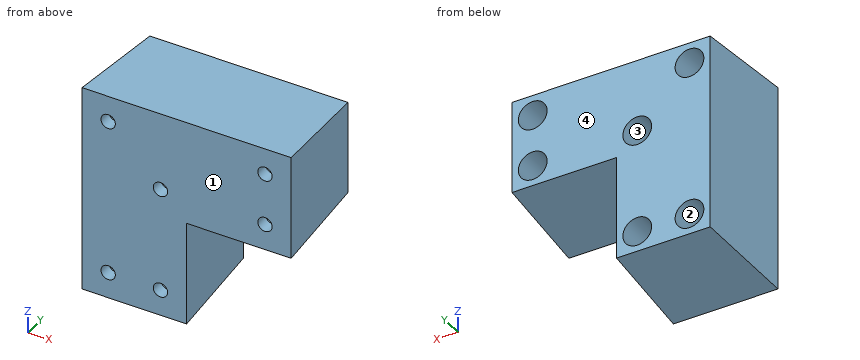
from build123d import *

# Parameters (mm, degrees)
BOSS_EXTRUDE1_DEPTH             = 40
BOSS_EXTRUDE1_TAPER             = 3
CBORE_FOR_M5_SBHCS1_D           = 5.5
CBORE_FOR_M5_SBHCS1_CBORE_D     = 11
CBORE_FOR_M5_SBHCS1_CBORE_DEPTH = 35


with BuildPart() as part:
    # Sketch1 → Boss-Extrude1 (new body)
    with BuildSketch(Plane(origin=(0, 0, 0), x_dir=(1, 0, 0), z_dir=(0, 1, 0))):
        Polygon((0, 0), (80, 0), (80, 40), (40, 40), (40, 80), (0, 80), align=None)
    extrude(amount=BOSS_EXTRUDE1_DEPTH, taper=BOSS_EXTRUDE1_TAPER)

    # CBORE for M5 SBHCS1 (through all)
    with Locations(Plane(origin=(0, 40, 0), x_dir=(1, 0, 0), z_dir=(0, 1, 0))):
        with Locations((10, 70), (30, 70), (70, 30), (70, 10), (30, 30), (10, 10)):
            CounterBoreHole(CBORE_FOR_M5_SBHCS1_D / 2, CBORE_FOR_M5_SBHCS1_CBORE_D / 2, CBORE_FOR_M5_SBHCS1_CBORE_DEPTH)


solid = part.part
For this review, take the finished solid that the model builds, in its own axes (mm). Face numbers are marked on the shaded views. A direction names the side the tool comes from. Coordinates: 2 decimals unless noted, no trailing zeros. Write each question's results on one line, items separated by ' | '. Start each with the question number.
1) For the marked faces 3 and 4, list the 3-axis set-ups (+Z, -Z, +X, -X, +Y, -Y) from which the entire face can be reached by the end or side of a thin tool; tool diameter is ignored.
2) The part is to be moulded in two halves that separate along X. For the marked faces 1 and 2, say which applies: +X half, -X half, draft (parallel to the pull), parting line (faces both ways), or undercut.
3) Insertion check: pin 1 (4 mm diameter, centred on x = 58, z = -11, fed in from -Y); pin 2 (1 mm diameter, centred on x = 71, y = 19, fed in from -Z); pin 3 (10 mm diameter, centred on x = 70, z = -30, fed in from +Y); pin 4 (5 mm diameter, centred on x = 43.5, y = 12, fed in from +Z). Each pin has a flat end and moves straight along its axis. Give the tip position at first contact, or say it passes through.
4) Consider section A-A (x = 10). Give the number of separate pieces and of enclosed holes in the cut face, plus the area to 3 significant figures.
5) Wall thickness on L1, parallel to Z at x = 27, y = 14.5; L2, parallel to Z at x = 11, y = 3; L3, parallel to X at y = 35.5, z = -27: over which ranges is each line inside the solid? List them lowest first. Write a range as [from, to].
Geometry says:
1) face 3: +Y | face 4: +Z, -Z, +X, -X, +Y
2) face 1: draft | face 2: undercut
3) pin 1: y = 0 | pin 2: z = -39.03 | pin 3: y = 5 | pin 4: z = -0.5
4) separate pieces: 3 | enclosed holes: 0 | area: 2,290 mm^2
5) L1: [-79.24, -74.61], [-65.39, -34.61], [-25.39, -0.76] | L2: [-79.84, -72.56], [-67.44, -12.56], [-7.44, -0.16] | L3: [1.86, 25.39], [34.61, 65.39], [74.61, 78.14]
